from build123d import *

# Parameters (mm, degrees)
CYLINDER002_R     = 0.4
CYLINDER002_DEPTH = 3
CYLINDER001_R     = 0.4
CYLINDER001_DEPTH = 3
BOX001_W          = 1
BOX001_H          = 1
BOX001_DEPTH      = 4
BOX_W             = 1
BOX_H             = 1
BOX_DEPTH         = 4
TORUS_R           = 2
CYLINDER_R        = 9.25
CYLINDER_DEPTH    = 26.5
FILLET_R          = 0.5


with BuildPart() as pin2:
    # Cylinder002 → Cylinder002 (new body)
    with BuildSketch(Plane(origin=(3.75, 0, -3), x_dir=(1, 0, 0), z_dir=(0, 0, 1))):
        Circle(CYLINDER002_R)
    extrude(amount=CYLINDER002_DEPTH)


with BuildPart() as pin1:
    # Cylinder001 → Cylinder001 (new body)
    with BuildSketch(Plane(origin=(-3.75, 0, -3), x_dir=(1, 0, 0), z_dir=(0, 0, 1))):
        Circle(CYLINDER001_R)
    extrude(amount=CYLINDER001_DEPTH)


with BuildPart() as box001:
    # Box001 → Box001 (new body)
    with BuildSketch(Plane(origin=(9, -0.5, 17), x_dir=(1, 0, 0), z_dir=(0, 0, 1))):
        with Locations((0.5, 0.5)):
            Rectangle(BOX001_W, BOX001_H)
    extrude(amount=BOX001_DEPTH)


with BuildPart() as box:
    # Box → Box (new body)
    with BuildSketch(Plane(origin=(9, -0.5, 9), x_dir=(1, 0, 0), z_dir=(0, 0, 1))):
        with Locations((0.5, 0.5)):
            Rectangle(BOX_W, BOX_H)
    extrude(amount=BOX_DEPTH)


with BuildPart() as ring:
    # Torus → Torus (revolve)
    with BuildSketch(Plane(origin=(0, 0, 3.5), x_dir=(1, 0, 0), z_dir=(0, -1, 0))):
        with Locations((10.75, 0)):
            Circle(TORUS_R)
    revolve(axis=Axis((0, 0, 3.5), (0, 0, 1)))


with BuildPart() as obj1:
    # Cylinder → Cylinder (new body)
    with BuildSketch(Plane.XY):
        Circle(CYLINDER_R)
    extrude(amount=CYLINDER_DEPTH)

    # Fillet
    fillet_edges = [obj1.edges().sort_by_distance(p)[0] for p in [
        (-9.25, 0, 26.5),
        (-9.25, 0, 0),
    ]]
    fillet(fillet_edges, radius=FILLET_R)

    # Cut: cut Ring
    add(ring.part, mode=Mode.SUBTRACT)

    # Cut001: cut Box
    add(box.part, mode=Mode.SUBTRACT)

    # Cut002: cut Box001
    add(box001.part, mode=Mode.SUBTRACT)

    # Fusion: union Pin1+
    add(pin1.part)

    # Fusion001: union Pin2-
    add(pin2.part)


solid = obj1.part
The listing builds one solid part. Answer for the finished solid, in the listing's coordinates (mm). A direction names the side the tool comes from. Coordinates: 2 decimals unless noted, no trailing zeros. Loops run counter-clockwise (first coordinate to the right, second up) from the corner with the lowest first, then second, coordinate; pieces in that order, holes last. Notation, with made-up numbers: (79.25, 23.25) -> (109.25, 23.25) arc R32 cw to (109.25, 58.25) -> close; hole circle Ø6 at (60, -10.5). An arc over 180 degrees is marked (long way). Answer in a Markdown table with one row per item. Add a question column.
1. The part is cut by section D-D, the plane z = 15. Write down the section's boundary in (x, y), then the cut area to 3 significant figures.
2. The part is cut by section C-C, the plane z = 19.5. Write down the section's boundary in (x, y).
3. Flat-ended cylindrical pins translate along their axes: P1, Ø8, axis at y = 6, z = 10.5, coming from the +X side; P2, Ø10, axis at x = -2.5, y = -6, coming from the -Z side; P3, Ø1.1, axis at y = 0, z = 11, coming from the +X side. Find the tip coordinate at first contact, or state that the pin passes through.
4. For faces 1 (the flat face through (0, 0, 26.5)), 2 (the cylindrical face through (3.35, 0.02, -1.52)), 3 (the flat face through (9, 0, 11)), determine the directions among +Z, -Z, +X, -X, +Y, -Y from which every point of the face is accessible in a straight line to the end or side of a thin tool.
5. The part is cut by section B-B, the plane y = 0. Write down the section's boundary in (x, z), then the cut area to 3 significant figures.
6. The part is cut by section A-A, the plane x = 0. Write down the section's boundary in (y, z).
7. Consider line 1 (Z direction, x = 3.5, y = -6.25); line 2 (X direction, y = 3, z = 1.25); line 3 (Z direction, x = -7.25, y = 5.5). Determine where each line is inside the solid, lowest interval first. Write a range as [from, to].
8. Determine the mould class of faces 4 (the cylindrical face through (-4.15, 0.02, -1.52)), 5 (the cylindrical face through (-2.01, -9.03, 15.26)), 6 (the flat face through (9, 0, 19)) for opening direction X: +X half, -X half, draft (parallel to the pull), parting line (faces both ways), or undercut.
Answer below:
| question | item | result |
|---|---|---|
| 1 | outline | circle Ø18.5 at (0, 0) |
| 1 | area | 269 mm2 |
| 2 | outline | (9, -0.5) -> (9, 0.5) -> (9.24, 0.5) arc R9.25 ccw (long way) to (9.24, -0.5) -> close |
| 3 | P1 | x = 9.03 |
| 3 | P2 | z = 0 |
| 3 | P3 | x = 9.24 |
| 4 | face 1 | +Z, +X, -X, +Y, -Y |
| 4 | face 2 | -Z |
| 4 | face 3 | +X |
| 5 | outline | (-9.25, 0.5) arc R0.5 ccw to (-8.75, 0) -> (-4.15, 0) -> (-4.15, -3) -> (-3.35, -3) -> (-3.35, 0) -> (3.35, 0) -> (3.35, -3) -> (4.15, -3) -> (4.15, 0) -> (8.75, 0) arc R0.5 ccw to (9.25, 0.5) -> (9.25, 2.18) arc R2 cw to (9.25, 4.82) -> (9.25, 9) -> (9, 9) -> (9, 13) -> (9.25, 13) -> (9.25, 17) -> (9, 17) -> (9, 21) -> (9.25, 21) -> (9.25, 26) arc R0.5 ccw to (8.75, 26.5) -> (-8.75, 26.5) arc R0.5 ccw to (-9.25, 26) -> (-9.25, 4.82) arc R2 cw to (-9.25, 2.18) -> close |
| 5 | area | 491 mm2 |
| 6 | outline | (-9.25, 0.5) arc R0.5 ccw to (-8.75, 0) -> (8.75, 0) arc R0.5 ccw to (9.25, 0.5) -> (9.25, 2.18) arc R2 cw to (9.25, 4.82) -> (9.25, 26) arc R0.5 ccw to (8.75, 26.5) -> (-8.75, 26.5) arc R0.5 ccw to (-9.25, 26) -> (-9.25, 4.82) arc R2 cw to (-9.25, 2.18) -> close |
| 7 | line 1 | [0, 26.5] |
| 7 | line 2 | [-8.75, 8.75] |
| 7 | line 3 | [0.14, 2.37], [4.63, 26.36] |
| 8 | face 4 | undercut |
| 8 | face 5 | parting line |
| 8 | face 6 | +X half |
